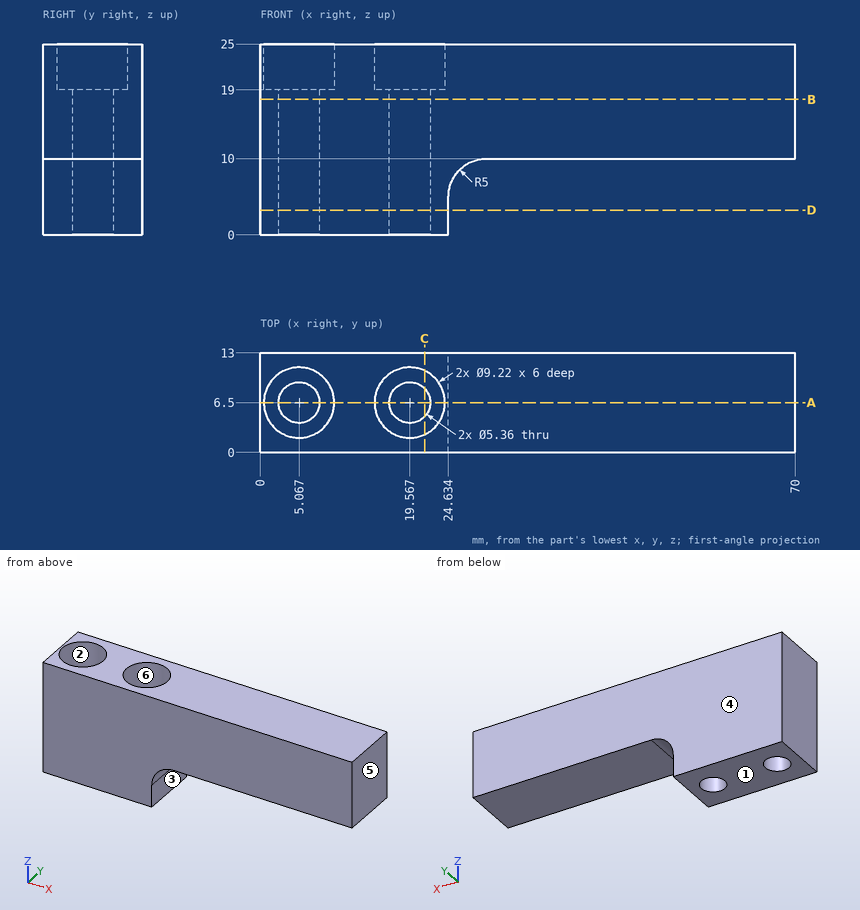
Here's the drawing with two shaded views (mm, measured from the low corner). I have some questions. A direction names the side the tool comes from. Coordinates: 2 decimals unless noted, no trailing zeros. Loops run counter-clockwise (first coordinate to the right, second up) from the corner with the lowest first, then second, coordinate; pieces in that order, holes last. Notation, with made-up numbers: (39.5, -1) -> (90.5, -1) arc R29 cw to (90.5, 30) -> close; hole circle Ø11 at (83.5, 32). An arc over 180 degrees is marked (long way). Answer as a JSON object with one key per item and string values.
1) For P1, Ø7.5, axis at x = 19.567, y = 6.5, coming from the +Z side; P2, Ø3, axis at x = 5.067, y = 6.5, coming from the -Z side; P3, Ø4, axis at y = 9, z = 3.5, coming from the +X side; P4, Ø4, axis at y = 10, z = 3, coming from the +X side, each with a flat end and sliding along its axis, tell me the tip position at first contact or that it passes through.
Results:
{"P1": "stops at z = 19", "P2": "passes through", "P3": "stops at x = 24.66", "P4": "stops at x = 24.63"}
2) If I drill on line 1 (X direction, y = 7.75, z = 12.75); line 2 (X direction, y = 7, z = 4); line 3 (Z direction, x = 63, y = 6.25), over which ranges is the centre line in solid material (lowest first)?
Results:
{"line 1": "x = 0 to 2.7, 7.44 to 17.2, 21.94 to 70", "line 2": "x = 0 to 2.43, 7.7 to 16.93, 22.2 to 24.63", "line 3": "z = 10 to 25"}
3) For the marked faces 1, 2 and 3, which set-ups out of +Z, -Z, +X, -X, +Y, -Y let a thin tool reach every point of the face, with its end or its side?
Results:
{"face 1": "-Z, +X, -X, +Y, -Y", "face 2": "+Z", "face 3": "-Z, +X, +Y, -Y"}
4) Imagine slicing it at D-D (z = 3.25). Please give me the cut outline in (x, y), then the cut area to 3 significant figures.
Results:
{"outline": "(0, 0) -> (24.63, 0) -> (24.63, 13) -> (0, 13) -> close; hole circle Ø5.36 at (5.07, 6.5); hole circle Ø5.36 at (19.57, 6.5)", "area": "275 mm^2"}
5) Imagine slicing it at A-A (y = 6.5). Please give me the cut outline in (x, z), then the cut area to 3 significant figures.
Results:
{"outline": "(0, 0) -> (2.39, 0) -> (2.39, 19) -> (0.46, 19) -> (0.46, 25) -> (0, 25) -> close; (7.75, 0) -> (16.89, 0) -> (16.89, 19) -> (14.96, 19) -> (14.96, 25) -> (9.68, 25) -> (9.68, 19) -> (7.75, 19) -> close; (22.25, 0) -> (24.63, 0) -> (24.63, 5) arc R5 cw to (29.63, 10) -> (70, 10) -> (70, 25) -> (24.18, 25) -> (24.18, 19) -> (22.25, 19) -> close", "area": "987 mm^2"}
6) Imagine slicing it at C-C (x = 21.5). Please give me the cut outline in (y, z), then the cut area to 3 significant figures.
Results:
{"outline": "(0, 0) -> (4.64, 0) -> (4.64, 19) -> (2.31, 19) -> (2.31, 25) -> (0, 25) -> close; (8.36, 0) -> (13, 0) -> (13, 25) -> (10.69, 25) -> (10.69, 19) -> (8.36, 19) -> close", "area": "204 mm^2"}
7) Imagine slicing it at B-B (z = 17.75). Please give me the cut outline in (x, y), then the cut area to 3 significant figures.
Results:
{"outline": "(0, 0) -> (70, 0) -> (70, 13) -> (0, 13) -> close; hole circle Ø5.36 at (5.07, 6.5); hole circle Ø5.36 at (19.57, 6.5)", "area": "865 mm^2"}
8) Thinking about a two-plate mould opening in Y: for the marked faces 4, 5 and 6, which applies, pulls with the +Y half, pulls with the -Y half, needs draft (parallel to the pull), parting line crosses it, or undercut?
Results:
{"face 4": "pulls with the +Y half", "face 5": "needs draft", "face 6": "undercut"}
